Input: dimensioned drawing with shaded views. Units: mm. Origin: part minimum x, y, z. Coordinates: 2 decimals unless noted, no trailing zeros. Write each loop counter-clockwise with the first axis right and the second up, starting at its lowest first coordinate (ties: lowest second). Pieces come first, ordered by that corner, then holes. Notation, with made-up numbers: M 15,-5.75 L 40,-5.75 A29 cw 40,29.25 Z; hole C -31,-25 d10. An arc over 180 degrees is marked long. Write each question's results on one line, items separated by ' | '. Start each with the question number.
1. Section query C-C, the plane x = 35. Output: boundary loops of the cut face in (y, z).
2. Section query A-A, the plane x = 60. Output: boundary loops of the cut face in (y, z).
3. Section query D-D, the plane z = 8. Output: boundary loops of the cut face in (x, y), and give its area (3 significant figures).
4. First-contact query: pin 1 (5 mm diameter, centred on x = 101, z = 5, fed in from +Y); pin 2 (1 mm diameter, centred on x = 13.5, z = 2, fed in from +Y); pin 3 (3 mm diameter, centred on x = 29.5, z = 4, fed in from +Y). Flat tips, straight axial feed; report the tip coordinate or a pass-through.
5. Pull-direction query (Y, two-part tool) for the marked faces 1, 2 and 3; classes: +Y half, -Y half, draft (parallel to the pull), parting line (faces both ways), or undercut.
6. Ray query, probe 1 along Y at (x, z) = (82, 4.25) (1 decimal); probe 2 along Y at (x, z) = (60, 2); probe 3 along Y at (x, z) = (35, 6.5) (1 decimal). Return the intervals inside material, ascending.
7. Section query B-B, the plane y = 60. Output: boundary loops of the cut face in (x, z), and give its area (3 significant figures).
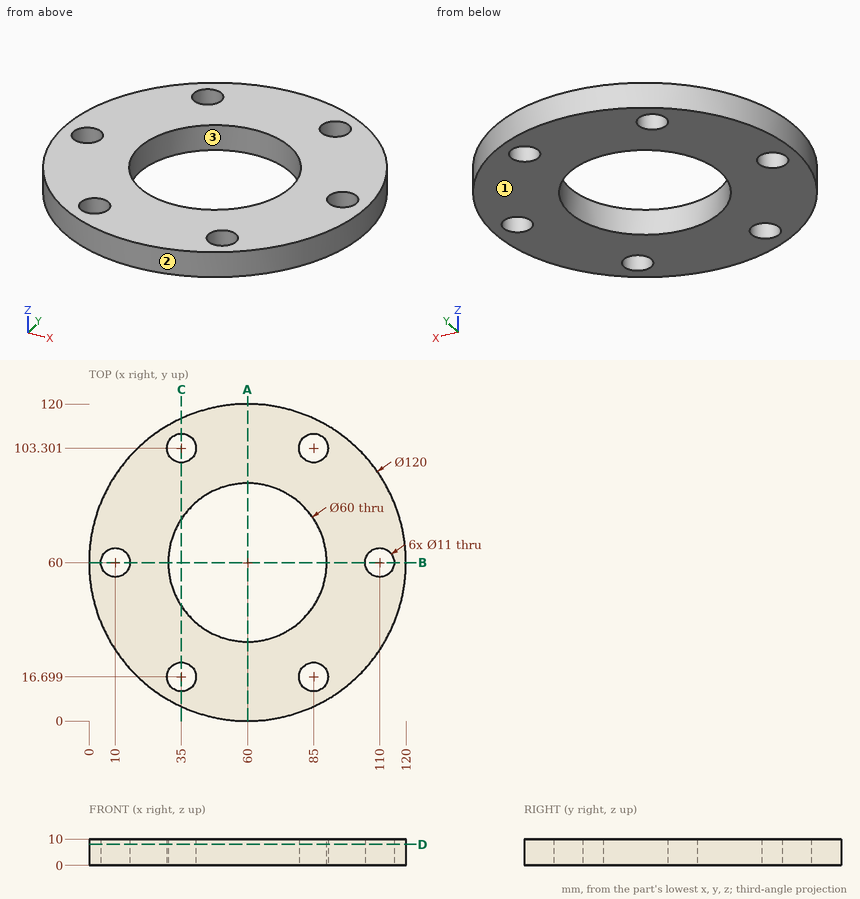
Answer:
1) outline: M 5.46,0 L 11.2,0 L 11.2,10 L 5.46,10 Z; M 22.2,0 L 43.42,0 L 43.42,10 L 22.2,10 Z; M 76.58,0 L 97.8,0 L 97.8,10 L 76.58,10 Z; M 108.8,0 L 114.54,0 L 114.54,10 L 108.8,10 Z
2) outline: M 0,0 L 30,0 L 30,10 L 0,10 Z; M 90,0 L 120,0 L 120,10 L 90,10 Z
3) outline: C 60,60 d120; hole C 10,60 d11; hole C 35,16.7 d11; hole C 35,103.3 d11; hole C 60,60 d60; hole C 85,16.7 d11; hole C 85,103.3 d11; hole C 110,60 d11 | area: 7,910 mm^2
4) pin 1: y = 106.02 | pin 2: y = 98.52 | pin 3: y = 112.53
5) face 1: draft | face 2: parting line | face 3: undercut
6) probe 1: 4.2 to 12.1, 21.3 to 39.6, 80.4 to 98.7, 107.9 to 115.8 | probe 2: 0 to 30, 90 to 120 | probe 3: 5.5 to 11.2, 22.2 to 43.4, 76.6 to 97.8, 108.8 to 114.5
7) outline: M 0,0 L 4.5,0 L 4.5,10 L 0,10 Z; M 15.5,0 L 30,0 L 30,10 L 15.5,10 Z; M 90,0 L 104.5,0 L 104.5,10 L 90,10 Z; M 115.5,0 L 120,0 L 120,10 L 115.5,10 Z | area: 380 mm^2
